Study the drawing (mm; zero at the part's minimum x, y, z) and answer. Give positions to 0.01 mm unless a question says otherwise; leave off trailing zeros. Order: outer loops, then holes, each group sorted by start corner. A loop starts at its lowest first (then second) coordinate and runs counter-clockwise, first axis right, second up. Notation, with made-up numbers: (4, -7.5) - (24, -7.5) arc R17 ccw to (24, 10.5) - close; hole circle Ø3 at (19, 6). An arc over 180 degrees is marked (long way). Return JSON: item names as keys, results as strings.
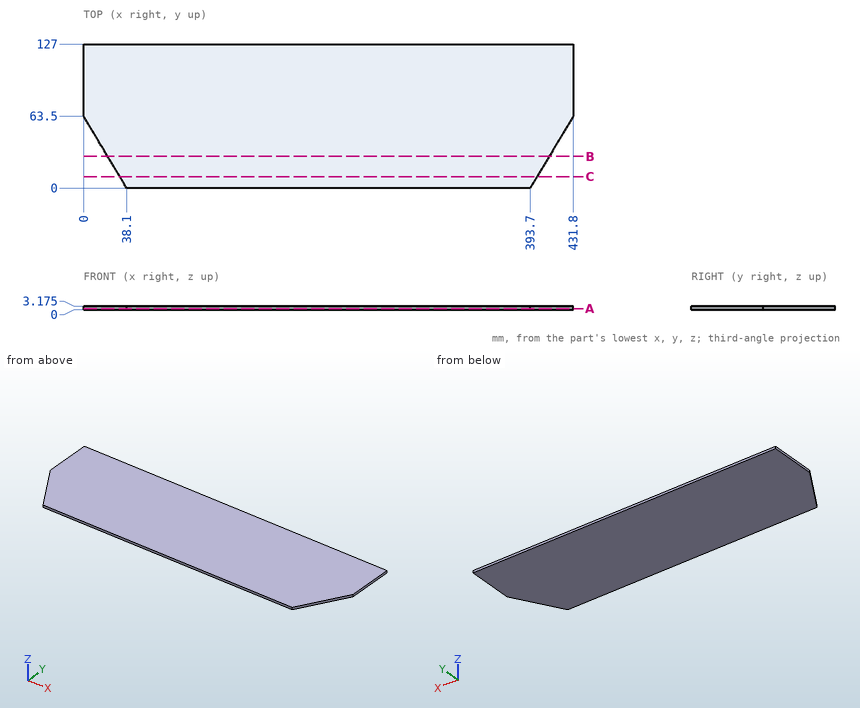
Q1. Consider L1, parallel to X at y = 29.5, z = 2.2; L2, parallel to X at y = 35, z = 2.9; L3, parallel to Y at x = 401, z = 1. Determine where each line is inside the solid, lowest interval first.
Values:
{"L1": "x = 20.4 to 411.4", "L2": "x = 17.1 to 414.7", "L3": "y = 12.17 to 127"}
Q2. A cutting plane is placed at A-A (z = 0.9). Write down the section's boundary in (x, y).
Values:
{"outline": "(0, 63.5) - (38.1, 0) - (393.7, 0) - (431.8, 63.5) - (431.8, 127) - (0, 127) - close"}
Q3. A cutting plane is placed at C-C (y = 10). Write down the section's boundary in (x, z) (3 decimals), and give its area (3 significant figures).
Values:
{"outline": "(32.1, 0) - (399.7, 0) - (399.7, 3.175) - (32.1, 3.175) - close", "area": "1,170 mm²"}
Q4. A cutting plane is placed at B-B (y = 28). Write down the section's boundary in (x, z) (3 decimals), and give its area (3 significant figures).
Values:
{"outline": "(21.3, 0) - (410.5, 0) - (410.5, 3.175) - (21.3, 3.175) - close", "area": "1,240 mm²"}
